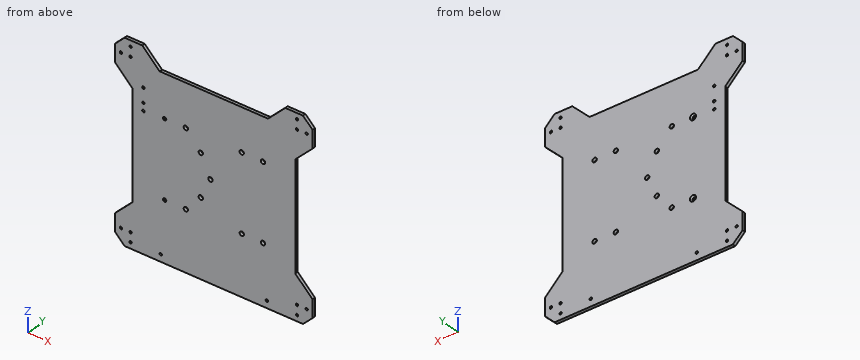
from build123d import *

# Parameters (mm, degrees)
BOSS_EXTRUDE1_DEPTH                             = 3.175
SKETCH2_R                                       = 1.5
SKETCH2_R_2                                     = 2.25
CUT_EXTRUDE1_DEPTH                              = 4.175
M3X0_5_TAPPED_HOLE1_D                           = 2.5
SKETCH5_R                                       = 1.25
CUT_EXTRUDE2_DEPTH                              = 4.175
SKETCH6_R                                       = 1.25
CUT_EXTRUDE3_DEPTH                              = 10
CSK_FOR_M3_FLAT_HEAD_MACHINE_SCREW1_D           = 3.4
CSK_FOR_M3_FLAT_HEAD_MACHINE_SCREW1_CSINK_D     = 6.3
CSK_FOR_M3_FLAT_HEAD_MACHINE_SCREW1_CSINK_ANGLE = 90
CUT_EXTRUDE4_DEPTH                              = 10


with BuildPart() as part:
    # Sketch1 → Boss-Extrude1 (new body)
    with BuildSketch(Plane(origin=(0, 0, 0), x_dir=(1, 0, 0), z_dir=(0, 1, 0))):
        Polygon((-92.5, 102.5), (92.5, 102.5), (102.5, 92.5), (102.5, -92.5), (92.5, -102.5), (-92.5, -102.5), (-102.5, -92.5), (-102.5, 92.5), align=None)
    extrude(amount=BOSS_EXTRUDE1_DEPTH)

    # Sketch2 → Cut-Extrude1 (cut, through all)
    with BuildSketch(Plane(origin=(0, 3.175, 0), x_dir=(1, 0, 0), z_dir=(0, 1, 0))):
        with Locations(Location((-51, -40, 0), (0, 0, 270))):  # turned: the seam where the file's is
            Circle(SKETCH2_R)
        with Locations(Location((-29, -40, 0), (0, 0, 270))):  # turned: the seam where the file's is
            Circle(SKETCH2_R_2)
        with Locations(Location((-51, 40, 0), (0, 0, 270))):  # turned: the seam where the file's is
            Circle(SKETCH2_R)
        with Locations(Location((-29, 40, 0), (0, 0, 270))):  # turned: the seam where the file's is
            Circle(SKETCH2_R_2)
        with Locations(Location((29, 40, 0), (0, 0, 270))):  # turned: the seam where the file's is
            Circle(SKETCH2_R_2)
        with Locations(Location((51, 40, 0), (0, 0, 270))):  # turned: the seam where the file's is
            Circle(SKETCH2_R_2)
        with Locations(Location((29, -40, 0), (0, 0, 270))):  # turned: the seam where the file's is
            Circle(SKETCH2_R_2)
        with Locations(Location((51, -40, 0), (0, 0, 270))):  # turned: the seam where the file's is
            Circle(SKETCH2_R_2)
        with Locations(Location((-3.5, 0, 0), (0, 0, 270))):  # turned: the seam where the file's is
            Circle(SKETCH2_R_2)
        with Locations(Location((-13.5, 22, 0), (0, 0, 270))):  # turned: the seam where the file's is
            Circle(SKETCH2_R_2)
        with Locations(Location((-13.5, -22, 0), (0, 0, 270))):  # turned: the seam where the file's is
            Circle(SKETCH2_R_2)
    extrude(amount=-CUT_EXTRUDE1_DEPTH, mode=Mode.SUBTRACT)

    # M3x0.5 Tapped Hole1 (through all)
    with Locations(Plane(origin=(0, 3.175, 0), x_dir=(-1, 0, 0), z_dir=(0, 1, 0))):
        with Locations((96.3, -86.3), (86.3, -96.3), (-86.3, -96.3), (-96.3, -86.3), (-96.3, 86.3), (-86.3, 96.3), (86.3, 96.3), (96.3, 86.3), (-86.3, 86.3), (-86.3, -86.3), (86.3, -86.3), (86.3, 86.3)):
            Hole(M3X0_5_TAPPED_HOLE1_D / 2)

    # Sketch5 → Cut-Extrude2 (cut, through all)
    with BuildSketch(Plane(origin=(0, 3.175, 0), x_dir=(1, 0, 0), z_dir=(0, 1, 0))):
        with Locations(Location((-55, 95, 0), (0, 0, 270))):  # turned: the seam where the file's is
            Circle(SKETCH5_R)
        with Locations(Location((55, 95, 0), (0, 0, 270))):  # turned: the seam where the file's is
            Circle(SKETCH5_R)
        with Locations(Location((-55, -95, 0), (0, 0, 270))):  # turned: the seam where the file's is
            Circle(SKETCH5_R)
        with Locations(Location((55, -95, 0), (0, 0, 270))):  # turned: the seam where the file's is
            Circle(SKETCH5_R)
    extrude(amount=-CUT_EXTRUDE2_DEPTH, mode=Mode.SUBTRACT)

    # Sketch6 → Cut-Extrude3 (cut)
    with BuildSketch(Plane(origin=(0, 3.175, 0), x_dir=(1, 0, 0), z_dir=(0, 1, 0))):
        with Locations(Location((-73, -46.5, 0), (0, 0, 270))):  # turned: the seam where the file's is
            Circle(SKETCH6_R)
        with Locations(Location((-73, -38.5, 0), (0, 0, 270))):  # turned: the seam where the file's is
            Circle(SKETCH6_R)
        with Locations(Location((-73, -61.5, 0), (0, 0, 270))):  # turned: the seam where the file's is
            Circle(SKETCH6_R)
    extrude(amount=-CUT_EXTRUDE3_DEPTH, mode=Mode.SUBTRACT)

    # CSK for M3 Flat Head Machine Screw1 (through all)
    with Locations(Plane(origin=(0, 3.175, 0), x_dir=(-1, 0, 0), z_dir=(0, 1, 0))):
        with Locations((51, -40), (51, 40)):
            CounterSinkHole(CSK_FOR_M3_FLAT_HEAD_MACHINE_SCREW1_D / 2, CSK_FOR_M3_FLAT_HEAD_MACHINE_SCREW1_CSINK_D / 2, counter_sink_angle=CSK_FOR_M3_FLAT_HEAD_MACHINE_SCREW1_CSINK_ANGLE)

    # Sketch9 → Cut-Extrude4 (cut)
    with BuildSketch(Plane(origin=(0, 3.175, 0), x_dir=(1, 0, 0), z_dir=(0, 1, 0))):
        Polygon((-102.5, 74.215728753), (-84.5, 56.215728753), (-84.5, -56.215728753), (-102.5, -74.215728753), align=None)
        Polygon((102.5, 74.215728753), (84.5, 56.215728753), (84.5, -56.215728753), (102.5, -74.215728753), align=None)
        Polygon((-74.215728753, -102.5), (-56.215728753, -84.5), (56.215728753, -84.5), (74.215728753, -102.5), align=None)
    extrude(amount=-CUT_EXTRUDE4_DEPTH, mode=Mode.SUBTRACT)


solid = part.part
Part model, mm, in its own coordinate system. Round coordinates to 2 decimals unless told otherwise and drop trailing zeros. Write each loop counter-clockwise with the first axis right and the second up, starting at its lowest first coordinate (ties: lowest second). Pieces come first, ordered by that corner, then holes. Notation, with made-up numbers: M 1,37 L 50,37 A15 cw 50,43 Z; hole C 87.25,-11.75 d5. An arc over 180 degrees is marked long. Return JSON: item names as keys, results as strings. Group by question number.
(1) Drill centre lines: probe 1 along X at (y, z) = (2.2, -86.3); probe 2 along Z at (x, y) = (-86.3, 1.8); probe 3 along X at (y, z) = (1.8, -96.3). Where is each one in solid material? Low to high.
(2) Saw through at B-B on x = -45. Write the cut outline in (y, z) (3 decimals), then the cut area to 3 significant figures.
(3) Saw through at A-A on y = 0.65. Count the separate pieces of the cut face and the enclosed holes in it, then the cut area to 3 significant figures.
(4) Pin check, flat tip, straight feed: pin 1 Ø2 at (x, z) = (96.3, -86.3) entering from +Y. Stop position of the tip, or through.
(5) Saw through at C-C on z = 16. Write the cut outline in (x, y) (3 decimals), then the cut area to 3 significant figures.
Returned:
{
 "1": {"probe 1": "-102.5 to -97.55, -95.05 to -87.55, -85.05 to 85.05, 87.55 to 95.05, 97.55 to 102.5", "probe 2": "-102.5 to -97.55, -95.05 to -87.55, -85.05 to -58.02, 58.02 to 85.05, 87.55 to 95.05, 97.55 to 102.5", "probe 3": "-98.7 to -87.55, -85.05 to 85.05, 87.55 to 98.7"},
 "2": {"outline": "M 0,-102.5 L 3.175,-102.5 L 3.175,84.5 L 0,84.5 Z", "area": "594 mm²"},
 "3": {"separate pieces": "1", "enclosed holes": "28", "area": "34,500 mm²"},
 "4": {"pin 1": "through"},
 "5": {"outline": "M -84.5,0 L 84.5,0 L 84.5,3.175 L -84.5,3.175 Z", "area": "537 mm²"}
}
